CAD build for the part. Positions are in the model's coordinates, mm. A direction names the side the tool comes from. Give positions to 0.01 mm unless a question says otherwise; leave off trailing zeros. Order: outer loops, then holes, each group sorted by start corner. A loop starts at its lowest first (then second) coordinate and runs counter-clockwise, first axis right, second up. Notation, with made-up numbers: M 46,82.25 L 94,82.25 A20 ccw 94,109.25 Z; hole C 24.5,-23.75 d1. An arc over 180 degrees is marked long. Put each result on its own line as item: value. Start each with the question number.
1) Cut at D-D (y = 18.5). Write the cut outline in (x, z), and give its area (3 significant figures).
2) Two-plate mould, pull along Y, no slides. Class faces 4 (the face through (-15.14, 20.06, 2.9)), 5 (the face through (-17, -25, 11)), 6 (the face through (-17, 25, 10)), 7 (the face through (17, 0, 1)): released by +Y, released by -Y, zero draft, split by the parting line, or undercut.
3) Cut at B-B (y = 7). Write the cut outline in (x, z), and give its area (3 significant figures).
4) Drill centre lines: line 1 (Y direction, x = -9, z = 1.3); line 2 (Z direction, x = -19, y = 14); line 3 (X direction, y = -19.5, z = 8). Where is each one in solid material? Low to high. Write a range as [from, to].
5) Cut at C-C (x = -9). Write the cut outline in (y, z), and give its area (3 significant figures).
6) Cut at A-A (z = 23). Write the cut outline in (x, y), and give its area (3 significant figures).
7) Tool access for faces 1 (the face through (-16, 20, 18)), 2 (the face through (6, -0.6, 1)), 3 (the face through (-18, 15.25, 17)): list every direction of +Z, -Z, +X, -X, +Y, -Y with a clear straight run to the whole face (end or side of a thin tool).
8) Pin check, flat tips, straight feed: pin 1 (5 mm diameter, centred on x = -9, y = -7, fed in from +Z); pin 2 (3 mm diameter, centred on y = 19.5, z = 24.5, fed in from +X). Stop position of each tip, or through.
Autodesk Fusion 360 part; units mm, degrees
sketch "Sketch1" plane through (0, 0, 0) normal (0, 0, 1) x (1, 0, 0)
  line L0 (21, -25) -> (-21, -25)
  line L1 (-21, -25) -> (-21, 25)
  line L2 (-21, 25) -> (21, 25)
  line L3 (21, 25) -> (21, -25)
  line L4 (21, -25) -> (-21, 25) construction
  line L5 (-21, -25) -> (21, 25) construction
  line L6 (-21, 0) -> (-9, 0) construction
  line L7 (-9, 0) -> (-9, -7) construction
  line L8 (-9, -7) -> (-21, -7) construction
  line L9 (-21, -7) -> (-21, 0) construction
  line L10 (-21, 0) -> (-9, 0) construction
  line L11 (-9, 0) -> (-9, 7) construction
  line L12 (-9, 7) -> (-21, 7) construction
  line L13 (-21, 7) -> (-21, 0) construction
  circle A0 centre (-9, 7) radius 4.2
  circle A1 centre (-9, -7) radius 4.2
  line L14 (-21, 0) -> (6, 0) construction
  line L15 (17, -0.6) -> (-5, -0.6)
  line L16 (-5, -0.6) -> (-5, 0.6)
  line L17 (-5, 0.6) -> (17, 0.6)
  line L18 (17, 0.6) -> (17, -0.6)
  line L19 (17, -0.6) -> (-5, 0.6) construction
  line L20 (-5, -0.6) -> (17, 0.6) construction
  point P0 (6, 0)
  dimension "d1" = 42
  dimension "d2" = 50
  dimension "d3" = 12
  dimension "d4" = 7
  dimension "d5" = 12
  dimension "d6" = 7
  dimension "d7" = 8.4
  dimension "d8" = 8.4
  dimension "d9" = 27
  dimension "d10" = 22
  dimension "d11" = 1.2
extrude "Extrude1" add sketch "Sketch1" along normal blind 2 makes body 1
sketch "Sketch2" plane through (0, 0, 2) normal (0, 0, 1) x (-1, 0, 0)
  line L0 (5, -0.6) -> (-17, -0.6)
  line L1 (-17, -0.6) -> (-17, 0.6)
  line L2 (-17, 0.6) -> (5, 0.6)
  line L3 (5, 0.6) -> (5, -0.6)
  circle A0 centre (9, 7) radius 4.2
  circle A1 centre (9, -7) radius 4.2
  line L4 (-21, -25) -> (21, -25)
  line L5 (21, -25) -> (21, 25)
  line L6 (21, 25) -> (-21, 25)
  line L7 (-21, 25) -> (-21, -25)
  line L8 (21, -25) -> (16, -25)
  line L9 (16, -25) -> (16, -15.25)
  line L10 (16, -15.25) -> (21, -15.25)
  line L11 (21, -15.25) -> (21, -25)
  line L12 (21, 25) -> (16, 25)
  line L13 (16, 25) -> (16, 15.25)
  line L14 (16, 15.25) -> (21, 15.25)
  line L15 (21, 15.25) -> (21, 25)
  dimension "d14" = 5
  dimension "d15" = 9.75
  dimension "d16" = 5
  dimension "d17" = 9.75
extrude "Extrude2" add sketch "Sketch2" along normal blind 30 contours L4 L5 L8 L9 L10 L11 | L5 L6 L12 L13 L14 L15 bodies 1
fillet "Fillet1" radius 3 2 edges at (-16, -20.125, 2) (-16, 20.125, 2) on bodies 1
copy_body "Body->Comp1" bodies 1 removing the originals makes body 2 in component "Slit"
component "Slit" placed x (1, 0, 0) y (0, 1, 0) z (0, 0, 1) at (0, 0, 0)
Solution:
1. outline: M -21,0 L 21,0 L 21,2 L -13,2 A3 cw -16,5 L -16,32 L -21,32 Z
1. area: 236 mm²
2. face 4: zero draft
2. face 5: released by -Y
2. face 6: released by +Y
2. face 7: undercut
3. outline: M -21,0 L -13.2,0 L -13.2,2 L -21,2 Z; M -4.8,0 L 21,0 L 21,2 L -4.8,2 Z
3. area: 67.2 mm²
4. line 1: [-25, -11.2], [-2.8, 2.8], [11.2, 25]
4. line 2: [0, 2]
4. line 3: [-21, -16]
5. outline: M -25,0 L -11.2,0 L -11.2,2 L -25,2 Z; M -2.8,0 L 2.8,0 L 2.8,2 L -2.8,2 Z; M 11.2,0 L 25,0 L 25,2 L 11.2,2 Z
5. area: 66.4 mm²
6. outline: M -21,-25 L -16,-25 L -16,-15.25 L -21,-15.25 Z; M -21,15.25 L -16,15.25 L -16,25 L -21,25 Z
6. area: 97.5 mm²
7. face 1: +Z, +X, +Y, -Y
7. face 2: +Z, -Z
7. face 3: +Z, +X, -X
8. pin 1: through
8. pin 2: x = -16
